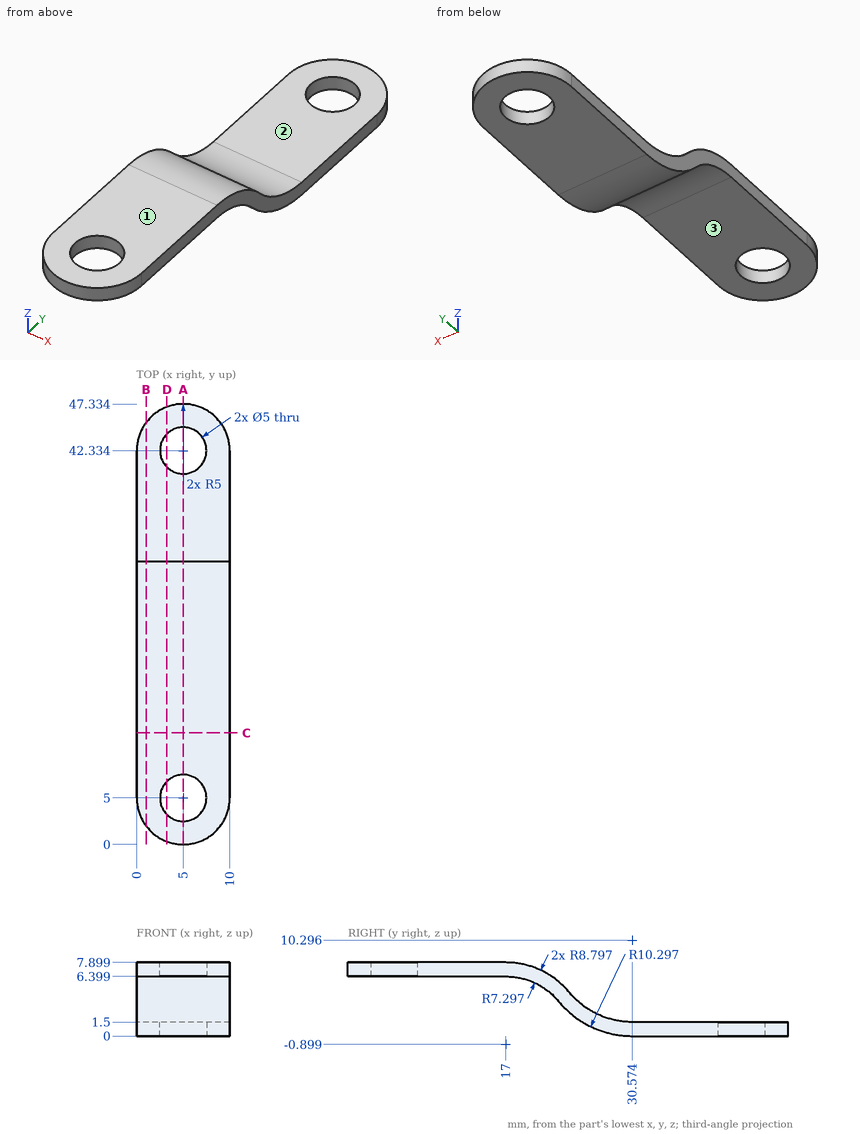
Answer from the drawing. Dimensions are ordinates in mm from the lowest x, y and z of the part. A direction names the side the tool comes from. Give positions to 0.01 mm unless a question says otherwise; leave off trailing zeros. Loops run counter-clockwise (first coordinate to the right, second up) from the corner with the lowest first, then second, coordinate; pieces in that order, holes last.
Item 1: The part is cut by section C-C (y = 12). Write down the section's boundary in (x, z).
Item 2: Each of these flat-tipped pins is pushed along its axis until it touches: pin 1 Ø4 at (y, z) = (39.5, 5) entering from +X; pin 2 Ø5 at (x, y) = (6.5, 7) entering from -Z; pin 3 Ø2 at (x, z) = (5.5, 3) entering from -Y; pin 4 Ø6 at (x, y) = (8.5, 29.5) entering from +Z. Where does it stop, or does it pass through?
Item 3: The part is cut by section B-B (x = 1). Write down the section's boundary in (y, z) (1 decimal).
Item 4: Find the intervals of material crossed by line 1 along Z through (x, y) = (1.5, 39); line 2 along Z through (x, y) = (7, 13); line 3 along Y through (x, z) = (5, 6.95) (1 decimal), in increasing order.
Item 5: For the marked faces 1, 2 and 3, determine the directions among +Z, -Z, +X, -X, +Y, -Y from which every point of the face is accessible in a straight line to the end or side of a thin tool.
Item 6: The part is cut by section A-A (x = 5). Write down the section's boundary in (y, z) (1 decimal).
Item 7: The part is cut by section D-D (x = 3.25). Write down the section's boundary in (y, z) (1 decimal).
Taken from the geometry:
1. outline: (0, 6.4) - (10, 6.4) - (10, 7.9) - (0, 7.9) - close
2. pin 1: passes through
2. pin 2: stops at z = 6.4
2. pin 3: stops at y = 22.41
2. pin 4: stops at z = 2.5
3. outline: (2, 6.4) - (17, 6.4) arc R7.3 cw to (22.6, 3.7) arc R10.3 ccw to (30.4, 0) - (45.3, 0) - (45.3, 1.5) - (30.4, 1.5) arc R8.8 cw to (23.8, 4.7) arc R8.8 ccw to (17, 7.9) - (2, 7.9) - close
4. line 1: z = 0 to 1.5
4. line 2: z = 6.4 to 7.9
4. line 3: y = 0 to 2.5, 7.5 to 21
5. face 1: +Z, +X, -X, +Y, -Y
5. face 2: +Z, +X, -X, +Y
5. face 3: -Z, +X, -X, -Y
6. outline: (0, 6.4) - (2.5, 6.4) - (2.5, 7.9) - (0, 7.9) - close; (7.5, 6.4) - (17, 6.4) arc R7.3 cw to (22.6, 3.7) arc R10.3 ccw to (30.4, 0) - (39.8, 0) - (39.8, 1.5) - (30.4, 1.5) arc R8.8 cw to (23.8, 4.7) arc R8.8 ccw to (17, 7.9) - (7.5, 7.9) - close; (44.8, 0) - (47.3, 0) - (47.3, 1.5) - (44.8, 1.5) - close
7. outline: (0.3, 6.4) - (3.2, 6.4) - (3.2, 7.9) - (0.3, 7.9) - close; (6.8, 6.4) - (17, 6.4) arc R7.3 cw to (22.6, 3.7) arc R10.3 ccw to (30.4, 0) - (40.5, 0) - (40.5, 1.5) - (30.4, 1.5) arc R8.8 cw to (23.8, 4.7) arc R8.8 ccw to (17, 7.9) - (6.8, 7.9) - close; (44.1, 0) - (47, 0) - (47, 1.5) - (44.1, 1.5) - close
